Design review of the part built by this model. Coordinates are the model's own, in mm. Give positions to 0.01 mm unless a question says otherwise; leave off trailing zeros. Order: outer loops, then holes, each group sorted by start corner. A loop starts at its lowest first (then second) coordinate and runs counter-clockwise, first axis right, second up. Notation, with made-up numbers: (2, 25) -> (19, 25) arc R20 cw to (19, 34) -> close; hole circle Ø5 at (-32.5, -16). An arc over 180 degrees is marked (long way). Answer in a Markdown table with one row per item. Add a question column.
```python
from build123d import *

# Parameters (mm, degrees)
SKETCH1_W               = 35
SKETCH1_H               = 55
SKETCH1_R               = 1.5
SKETCH1_W_2             = 1.053264104
SKETCH1_H_2             = 1.810086697
BOSS_EXTRUDE1_DEPTH     = 3
SKETCH2_W               = 30.130506089
SKETCH2_H               = 18.151203477
BOSS_EXTRUDE2_DEPTH     = 11
SKETCH4_W               = 25.972666726
SKETCH4_H               = 17.735623468
CUT_EXTRUDE2_DEPTH      = 4
CUT_EXTRUDE3_DEPTH      = 36.47534355
CUT_EXTRUDE3_DEPTH_BACK = 36.47534355
SKETCH6_R               = 1.5
CUT_EXTRUDE4_DEPTH      = 35.095454242
CUT_EXTRUDE4_DEPTH_BACK = 2.5
SKETCH7_R               = 3
SKETCH8_W               = 48.556860944
SKETCH8_H               = 13.798997775
CUT_EXTRUDE5_DEPTH      = 60.390655831


with BuildPart() as part:
    # Sketch1 → Boss-Extrude1 (new body)
    with BuildSketch(Plane(origin=(0, 0, 0), x_dir=(1, 0, 0), z_dir=(0, 1, 0))):
        Rectangle(SKETCH1_W, SKETCH1_H)
        with Locations(Location((12.5, 25, 0), (0, 0, 270))):
            Circle(SKETCH1_R, mode=Mode.SUBTRACT)
        with Locations(Location((-12.5, 25, 0), (0, 0, 270))):
            Circle(SKETCH1_R, mode=Mode.SUBTRACT)
        with Locations(Location((12.5, -25, 0), (0, 0, 270))):
            Circle(SKETCH1_R, mode=Mode.SUBTRACT)
        with Locations(Location((-12.5, -25, 0), (0, 0, 270))):
            Circle(SKETCH1_R, mode=Mode.SUBTRACT)
        with Locations((14.770586435, -21.896230663)):
            Rectangle(SKETCH1_W_2, SKETCH1_H_2, mode=Mode.SUBTRACT)
    extrude(amount=BOSS_EXTRUDE1_DEPTH)

    # Sketch2 → Boss-Extrude2 (add)
    with BuildSketch(Plane(origin=(0, 3, 0), x_dir=(1, 0, 0), z_dir=(0, 1, 0))):
        with Locations((1.371677436, 0.106547158)):
            Rectangle(SKETCH2_W, SKETCH2_H)
    extrude(amount=BOSS_EXTRUDE2_DEPTH)

    # Sketch4 → Cut-Extrude2 (cut)
    with BuildSketch(Plane.XZ):
        with Locations((1.214862274, -0.038232514)):
            Rectangle(SKETCH4_W, SKETCH4_H)
    extrude(amount=-CUT_EXTRUDE2_DEPTH, mode=Mode.SUBTRACT)

    # Sketch6 → Cut-Extrude3 (cut, two sides: drawn at the far end of the back side and taken through both)
    with BuildSketch(Plane.XZ.offset(-CUT_EXTRUDE3_DEPTH_BACK)):
        with Locations(Location((11.63, 3.25, 0), (0, 0, 270))):
            Circle(SKETCH6_R)
        with Locations(Location((-5.17, 5.05, 0), (0, 0, 270))):
            Circle(SKETCH6_R)
        with Locations(Location((-4.17, -3.15, 0), (0, 0, 270))):
            Circle(SKETCH6_R)
        with Locations(Location((6.33, -4.95, 0), (0, 0, 270))):
            Circle(SKETCH6_R)
    extrude(amount=CUT_EXTRUDE3_DEPTH + CUT_EXTRUDE3_DEPTH_BACK, mode=Mode.SUBTRACT)

    # Sketch7 → Cut-Extrude4 (cut, two sides: drawn at the far end of the back side and taken through both)
    with BuildSketch(Plane.XZ.offset(-4).offset(-CUT_EXTRUDE4_DEPTH_BACK)):
        with Locations(Location((-5.17, 5.05, 0), (0, 0, 90))):
            Circle(SKETCH7_R)
        with Locations(Location((-4.17, -3.15, 0), (0, 0, 90))):
            Circle(SKETCH7_R)
        with Locations(Location((6.33, -4.95, 0), (0, 0, 90))):
            Circle(SKETCH7_R)
        with Locations(Location((11.63, 3.25, 0), (0, 0, 31.011355011))):
            Circle(SKETCH7_R)
    extrude(amount=CUT_EXTRUDE4_DEPTH + CUT_EXTRUDE4_DEPTH_BACK, mode=Mode.SUBTRACT)

    # Sketch8 → Cut-Extrude5 (cut, through all)
    with BuildSketch(Plane.XY.offset(27.5)):
        with Locations((-0.01102719, 5.466634706)):
            Rectangle(SKETCH8_W, SKETCH8_H)
    extrude(amount=-CUT_EXTRUDE5_DEPTH, mode=Mode.SUBTRACT)


solid = part.part
```
1) Add section A-A, the plane z = 5.05. Write out the cut boundary in (x, y).
2) Add section C-C, the plane y = 13.3. Write out the cut boundary in (x, z).
3) Add section D-D, the plane x = -5.17. Write out the cut boundary in (y, z), and give its area (3 significant figures).
4) For L1, parallel to X at y = 13.3, z = -4.95; L2, parallel to X at y = 12.9, z = -3.15; L3, parallel to Z at x = 11.63, y = 13.65, list the stretches that pass through material, from the lowest coordinate up.
5) Add section B-B, the plane x = 11.63. Write out the cut boundary in (y, z), and give its area (3 significant figures).
6) Mouldability with a two-part tool opening along X and no side actions: class faces 1 (the face through (-2.683, 13.195, -2.955)), 2 (the face through (16.437, 13, 0)), 3 (the face through (1, 13, 8.969)) as +X half, -X half, draft (parallel to the pull), parting line (faces both ways), or undercut.
Verdict:
| question | item | result |
|---|---|---|
| 1 | outline | (-13.69, 12.37) -> (-6.67, 12.37) -> (-6.67, 14) -> (-13.69, 14) -> close; (-3.67, 12.37) -> (16.44, 12.37) -> (16.44, 14) -> (-3.67, 14) -> close |
| 2 | outline | (-13.69, -9.18) -> (16.44, -9.18) -> (16.44, 8.97) -> (-13.69, 8.97) -> close; hole circle Ø3 at (-5.17, 5.05); hole circle Ø3 at (-4.17, -3.15); hole circle Ø3 at (6.33, -4.95); hole circle Ø3 at (11.63, 3.25) |
| 3 | outline | (12.37, -9.18) -> (14, -9.18) -> (14, -4.27) -> (12.37, -4.27) -> close; (12.37, -2.03) -> (14, -2.03) -> (14, 3.55) -> (12.37, 3.55) -> close; (12.37, 6.55) -> (14, 6.55) -> (14, 8.97) -> (12.37, 8.97) -> close |
| 3 | area | 21.1 mm2 |
| 4 | L1 | x = -13.69 to 4.83, 7.83 to 16.44 |
| 4 | L2 | x = -13.69 to -5.67, -2.67 to 16.44 |
| 4 | L3 | z = -9.18 to 1.75, 4.75 to 8.97 |
| 5 | outline | (12.37, -9.18) -> (14, -9.18) -> (14, 1.75) -> (12.37, 1.75) -> close; (12.37, 4.75) -> (14, 4.75) -> (14, 8.97) -> (12.37, 8.97) -> close |
| 5 | area | 24.8 mm2 |
| 6 | face 1 | undercut |
| 6 | face 2 | +X half |
| 6 | face 3 | draft |
